For this review, take the finished solid that the model builds, in its own axes (mm). Round coordinates to 2 decimals unless told otherwise and drop trailing zeros. Write each loop counter-clockwise with the first axis right and the second up, starting at its lowest first coordinate (ties: lowest second). Pieces come first, ordered by that corner, then holes. Notation, with made-up numbers: M -24,83 L 5,83 A28 ccw 5,108 Z; hole C 9,31.5 d4. An arc over 180 degrees is marked long. One line per question, with ' | ' between items.
```python
from build123d import *

# Parameters (mm, degrees)
F0_W    = 7
F0_H    = 7
F2_R    = 0.75
F3_W    = 0.2
F3_H    = 5
F5_SIZE = 0.19999


# Not quite as in the source:
# - a fillet or chamfer is up to 0.001 mm smaller than in the source, because OpenCascade refuses the exact size


with BuildPart() as f1:
    # F0 (on Front) → F1 (revolve)
    with BuildSketch(Plane.XZ):
        with Locations((0, 7.5)):
            Rectangle(F0_W, F0_H)
    revolve(axis=Axis((-0.6671294104, 0, 0), (-1, 0, 0)))

    # F2
    f2_edges = [f1.edges().sort_by_distance(p)[0] for p in [
        (-3.5, 0, -11),
        (-3.5, 0, -4),
        (3.5, 0, -11),
        (3.5, 0, -4),
    ]]
    fillet(f2_edges, radius=F2_R)

    # F3 (on Top) → F4 (revolve, cut)
    with BuildSketch(Plane.XY):
        with Locations((-3.4, -7.5)):
            Rectangle(F3_W, F3_H)
        with Locations((3.4, -7.5)):
            Rectangle(F3_W, F3_H)
    revolve(axis=Axis((0.1337367576, 0, 0), (1, 0, 0)), mode=Mode.SUBTRACT)

    # F5 (size 0.2 in the source; OpenCascade refuses exactly that, so slightly less here)
    f5_edges = [f1.edges().sort_by_distance(p)[0] for p in [
        (-3.3, 10, 0),
        (-3.3, 5, 0),
        (3.3, 10, 0),
        (3.3, 5, 0),
    ]]
    chamfer(f5_edges, length=F5_SIZE)


solid = f1.part
```
Item 1: Insertion check: pin 1 Ø6 at (y, z) = (-1, 1) entering from +X; pin 2 Ø3 at (x, z) = (0.5, 2) entering from -Y; pin 3 Ø1.5 at (y, z) = (2, -7.5) entering from +X. Each pin has a flat end and moves straight along its axis. Give the tip position at first contact, or say it passes through.
Results:
pin 1: x = 3.42 | pin 2: y = -10.99 | pin 3: x = 3.3
Item 2: Mouldability with a two-part tool opening along Z and no side actions: class faces 1 (the face through (0.04, -10.74, -2.38)), 2 (the face through (3.3, -4, 4)), 3 (the face through (0.038, -3.905, -0.867)) as +Z half, -Z half, draft (parallel to the pull), parting line (faces both ways), or undercut.
Results:
face 1: parting line | face 2: undercut | face 3: undercut
Item 3: Take a section at A-A (x = -1.5). Write out the cut boundary in (y, z).
Results:
outline: C 0,0 d22; hole C 0,0 d8
Item 4: To check wall thickness, follow line 1 along X through (y, z) = (1.75, -8.5); line 2 along Y through (x, z) = (2.5, -2.5); line 3 along Y through (x, z) = (-2, -3.25). State the ranges of each line that lie inside material, in increasing order. Write a range as from..to.
Results:
line 1: -3.3..3.3 | line 2: -10.71..-3.12, 3.12..10.71 | line 3: -10.51..-2.33, 2.33..10.51
